```python
from build123d import *

# Parameters (mm, degrees)
CROQUIS1_W              = 29
CROQUIS1_H              = 40
SALIENTE_EXTRUIR1_DEPTH = 24.4
SALIENTE_EXTRUIR2_DEPTH = 1.6
CROQUIS3_R              = 5
CORTAR_EXTRUIR1_DEPTH   = 34


with BuildPart() as part:
    # Croquis1 → Saliente-Extruir1 (new body)
    with BuildSketch(Plane.XY):
        Rectangle(CROQUIS1_W, CROQUIS1_H)
    extrude(amount=SALIENTE_EXTRUIR1_DEPTH)

    # Croquis2 → Saliente-Extruir2 (add)
    with BuildSketch(Plane.XY):
        Polygon((14.5, 20), (32.5, 20), (32.5, -16.3), (24.5, -20), (14.5, -20), (14.5, -7), (21.5, -7), (27.5, 0), (27.5, 11), (14.5, 11), align=None)
    extrude(amount=SALIENTE_EXTRUIR2_DEPTH)

    # Croquis3 → Cortar-Extruir1 (cut)
    with BuildSketch(Plane.XZ.offset(20)):
        with Locations(Location((0, 13, 0), (0, 0, 270))):
            Circle(CROQUIS3_R)
    extrude(amount=-CORTAR_EXTRUIR1_DEPTH, mode=Mode.SUBTRACT)


solid = part.part
```
Geometry: final body of the model. Coordinates: model frame, mm. A direction names the side the tool comes from. Coordinates: 2 decimals unless noted, no trailing zeros. Loops run counter-clockwise (first coordinate to the right, second up) from the corner with the lowest first, then second, coordinate; pieces in that order, holes last. Notation, with made-up numbers: (-28, 56.5) -> (-22, 56.5) arc R6 cw to (-22, 66.5) -> close; hole circle Ø1 at (-39, 65.5). An arc over 180 degrees is marked (long way). Use a Markdown table: item, result. Add a question column.
(1) Section query C-C, the plane y = -8. Return loops of the section in (x, z), plus the area to 3 significant figures.
(2) Pin query (flat end, axial travel): pin 1 Ø3 at (x, z) = (-1, 11.5) entering from -Y; pin 2 Ø9 at (x, y) = (25.5, 3.5) entering from +Z; pin 3 Ø12 at (y, z) = (-10.5, 8) entering from +X. Return the tip coordinate at first contact, or that it passes through.
(3) Line query: line 1 along X through (y, z) = (-12.5, 13); line 2 along Z through (x, y) = (28.5, -2.5); line 3 along X through (y, z) = (1.5, 19.5). Output: solid intervals per line, ascending.
(4) Section query D-D, the plane z = 13. Return loops of the section in (x, y).
(5) Section query A-A, the plane y = 2. Return loops of the section in (x, z), plus the area to 3 significant figures.
(6) Mould query, pull axis Z, two halves, no side actions, for faces 1 (the flat face through (-14.5, 0, 12)), 2 (the cylindrical face through (1.5, -3.24, 8.23)), 3 (the flat face through (0, 14, 13)), 4 (the flat face through (9, 0, 0)). Classes: pulls with the +Z half, pulls with the -Z half, needs draft (parallel to the pull), parting line crosses it, or undercut.
(7) Access query for faces 5 (the flat face through (28, 0, 1.6)), 6 (the flat face through (0, 0, 24.4)), 7 (the flat face through (24.5, -3.5, 0.8)). Directions: +Z, -Z, +X, -X, +Y, -Y. A direction counts if a zero-diameter tool reaches every point of the face in a straight line with its end or side. Return the directions, or none.
(8) Section query B-B, the plane x = 17.5. Return loops of the section in (y, z), plus the area to 3 significant figures.
Answer:
| question | item | result |
|---|---|---|
| 1 | outline | (-14.5, 0) -> (32.5, 0) -> (32.5, 1.6) -> (14.5, 1.6) -> (14.5, 24.4) -> (-14.5, 24.4) -> close; hole circle Ø10 at (0, 13) |
| 1 | area | 658 mm^2 |
| 2 | pin 1 | stops at y = 14 |
| 2 | pin 2 | stops at z = 1.6 |
| 2 | pin 3 | stops at x = 14.5 |
| 3 | line 1 | x = -14.5 to -5, 5 to 14.5 |
| 3 | line 2 | z = 0 to 1.6 |
| 3 | line 3 | x = -14.5 to 14.5 |
| 4 | outline | (-14.5, -20) -> (-5, -20) -> (-5, 14) -> (5, 14) -> (5, -20) -> (14.5, -20) -> (14.5, 20) -> (-14.5, 20) -> close |
| 5 | outline | (-14.5, 0) -> (14.5, 0) -> (14.5, 24.4) -> (-14.5, 24.4) -> close; (27.5, 0) -> (32.5, 0) -> (32.5, 1.6) -> (27.5, 1.6) -> close; hole circle Ø10 at (0, 13) |
| 5 | area | 637 mm^2 |
| 6 | face 1 | needs draft |
| 6 | face 2 | undercut |
| 6 | face 3 | undercut |
| 6 | face 4 | pulls with the -Z half |
| 7 | face 5 | +Z, +X, +Y, -Y |
| 7 | face 6 | +Z, +X, -X, +Y, -Y |
| 7 | face 7 | +Z, -Z |
| 8 | outline | (-20, 0) -> (-7, 0) -> (-7, 1.6) -> (-20, 1.6) -> close; (11, 0) -> (20, 0) -> (20, 1.6) -> (11, 1.6) -> close |
| 8 | area | 35.2 mm^2 |
